The model under review builds one solid part; all positions refer to its coordinate system, in mm. Face numbers are marked on the shaded views. Coordinates: 2 decimals unless noted, no trailing zeros. Order: outer loops, then holes, each group sorted by start corner. A loop starts at its lowest first (then second) coordinate and runs counter-clockwise, first axis right, second up. Notation, with made-up numbers: M 62,-5 L 90,-5 A15 cw 90,7 Z; hole C 41.5,62.5 d5. An arc over 180 degrees is marked long. Answer as CSV lines item,"result". Start each with the question number.
Q1. Consider section A-A on y = 0. Write out the cut boundary in (x, z), and give its area (3 significant figures).
Q2. For P1, Ø1.5, axis at x = 16.5, y = -4, coming from the -Z side; P2, Ø3, axis at y = -9, z = 4, coming from the -X side, all flat-tipped, find the tip position at first contact; note any pin that passes through.
Q3. Wall thickness on L1, parallel to Y at x = 18, z = 3.4; L2, parallel to Y at x = 20, z = 1.05; L3, parallel to Y at x = 47, z = 0.55: over which ranges is each line inside the solid? List them lowest first. Write a range as [from, to].
Q4. Consider section D-D on y = -9. Write out the cut boundary in (x, z), and give its area (3 significant figures).
Q5. The part is to be moulded in two halves that separate along X. For the marked faces 1, 2, 3 and 4, say which applies: +X half, -X half, draft (parallel to the pull), parting line (faces both ways), or undercut.
Q6. Consider section C-C on z = 2.8. Write out the cut boundary in (x, y).
Q7. Consider section B-B on x = 19.5. Write out the cut boundary in (y, z), and give its area (3 significant figures).
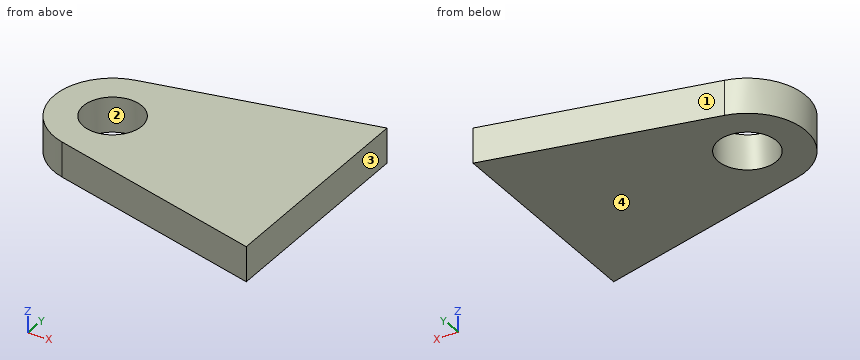
Autodesk Inventor part; units mm, degrees
ref_plane "YZ Plane" through (0, 0, 0) normal (1, 0, 0) x (0, 1, 0)
ref_plane "XZ Plane" through (0, 0, 0) normal (0, 1, 0) x (-1, 0, 0)
ref_plane "XY Plane" through (0, 0, 0) normal (0, 0, 1) x (1, 0, 0)
sketch "Sketch1" plane through (0, 0, 0) normal (0, 0, 1) x (1, 0, 0)
  circle A0 centre (-790.1228, -10.9134) radius 9.525
  ellipse E0 centre (61.5218, 18.65) end of major axis (52.5416, 18.65) minor radius 6.35 (61.5218, 25) -> (52.5416, 18.65) ccw
  line L0 (61.5218, 25) -> (114.272, 25)
  ellipse E1 centre (114.272, 18.65) end of major axis (105.2917, 18.65) minor radius 6.35 (123.2522, 18.65) -> (114.272, 25) ccw
  line L1 (123.2522, 18.65) -> (123.2522, -18.65)
  ellipse E2 centre (114.272, -18.65) end of major axis (105.2917, -18.65) minor radius 6.35 (114.272, -25) -> (123.2522, -18.65) ccw
  line L2 (114.272, -25) -> (61.5218, -25)
  ellipse E3 centre (61.5218, -18.65) end of major axis (52.5416, -18.65) minor radius 6.35 (52.5416, -18.65) -> (61.5218, -25) ccw
  line L3 (52.5416, -18.65) -> (52.5416, 18.65)
  line L4 (114.272, 21.825) -> (61.5218, 21.825)
  ellipse E4 centre (61.5218, 18.65) end of major axis (57.0317, 18.65) minor radius 3.175 (61.5218, 21.825) -> (57.0317, 18.65) ccw
  line L5 (57.0317, 18.65) -> (57.0317, -18.65)
  ellipse E5 centre (61.5218, -18.65) end of major axis (57.0317, -18.65) minor radius 3.175 (57.0317, -18.65) -> (61.5218, -21.825) ccw
  line L6 (61.5218, -21.825) -> (114.272, -21.825)
  ellipse E6 centre (114.272, -18.65) end of major axis (109.7818, -18.65) minor radius 3.175 (114.272, -21.825) -> (118.7621, -18.65) ccw
  line L7 (118.7621, -18.65) -> (118.7621, 18.65)
  ellipse E7 centre (114.272, 18.65) end of major axis (109.7818, 18.65) minor radius 3.175 (118.7621, 18.65) -> (114.272, 21.825) ccw
  circle A1 centre (17.6912, 0) radius 5
  circle A2 centre (17.6912, 0) radius 10
  line L8 (15.357, 9.7238) -> (52.5416, 18.65)
  line L9 (52.5416, -18.65) -> (15.357, -9.7238)
  dimension "d4" = 20
extrude "Extrusion1" add sketch "Sketch1" along normal blind 6 contours L3 L9 A2 L8 | A2
properties part number "Soporte pivote freno"
Evaluation:
1,outline,"M 7.69,0 L 12.69,0 L 12.69,6 L 7.69,6 Z; M 22.69,0 L 52.54,0 L 52.54,6 L 22.69,6 Z"
1,area,"209 mm²"
2,P1,"passes through"
2,P2,"stops at x = 11.08"
3,L1,"y = [-10.36, -4.99], [4.99, 10.36]"
3,L2,"y = [-10.84, -4.44], [4.44, 10.84]"
3,L3,"y = [-17.32, 17.32]"
4,outline,"M 13.33,0 L 52.54,0 L 52.54,6 L 13.33,6 Z"
4,area,"235 mm²"
5,face 1,"-X half"
5,face 2,"undercut"
5,face 3,"+X half"
5,face 4,"draft"
6,outline,"M 15.36,-9.72 L 52.54,-18.65 L 52.54,18.65 L 15.36,9.72 A10 ccw Z; hole C 17.69,0 d10"
7,outline,"M -10.72,0 L -4.66,0 L -4.66,6 L -10.72,6 Z; M 4.66,0 L 10.72,0 L 10.72,6 L 4.66,6 Z"
7,area,"72.7 mm²"
